The listing builds one solid part. Answer for the finished solid, in the listing's coordinates (mm). A direction names the side the tool comes from. Give positions to 0.01 mm unless a question says otherwise; leave off trailing zeros. Loops run counter-clockwise (first coordinate to the right, second up) from the corner with the lowest first, then second, coordinate; pieces in that order, holes last.
Item 1: Each of these flat-tipped pins is pushed along its axis until it touches: pin 1 Ø4 at (x, z) = (-17.5, -22) entering from +Y; pin 2 Ø1.5 at (x, z) = (7, -1) entering from -Y; pin 3 Ø6 at (x, z) = (-11.5, -0.5) entering from +Y. Where does it stop, or does it pass through?
Item 2: Section B-B, the plane z = -33 is taken. Give the vertices of the cut face in (x, y).
Item 3: A tool of negligible diameter and unlimited length cuts with its end or side. For faces 3 (the face through (-1, 10, -37)), 4 (the face through (38, -4, 29)), 5 (the face through (0.5, 9, -23)), 6 (the face through (39, 6, -33)), 7 (the face through (39, 4, 31)), from which of +Z, -Z, +X, -X, +Y, -Y can it reach the whole face along a straight path? Write none if from no direction.
Item 4: Section A-A, the plane y = 10.5 is taken. Give the number of separate pieces and of enclosed holes in the cut face, and give its area (3 significant figures).
Item 5: The mould has two halves that part along X. Classify faces 1 (the face through (-37, -4, -35)), 2 (the face through (-38.52, -3.93, 31.5)): pulls with the +X half, pulls with the -X half, needs draft (parallel to the pull), parting line crosses it, or undercut.
Item 6: Section D-D, the plane y = 19 is taken. Give the vertices of the cut face in (x, z), and give its area (3 significant figures).
Item 7: Consider line 1 along X through (y, z) = (2.5, 18); line 2 along X through (y, z) = (16.25, 31.5); line 3 along X through (y, z) = (20.25, -8). Determine where each line is inside the solid, lowest interval first.
from build123d import *

# Parameters (mm, degrees)
SKETCH_1_W          = 80
SKETCH_1_H          = 74
EXTRUDE_1_DEPTH     = 2
SKETCH_2_W          = 80
SKETCH_2_H          = 74
SKETCH_2_W_2        = 76
SKETCH_2_H_2        = 70
EXTRUDE_2_DEPTH     = 20
SKETCH_3_W          = 2
SKETCH_3_H          = 4
CUT_EXTRUDE_3_DEPTH = 4
SKETCH_4_W          = 1
SKETCH_4_H          = 16
SKETCH_4_H_2        = 20
EXTRUDE_3_DEPTH     = 15
SKETCH_6_W          = 3
SKETCH_6_H          = 8
EXTRUDE_4_DEPTH     = 8
SKETCH_7_R          = 1.5
CUT_EXTRUDE_5_DEPTH = 91.846023578


with BuildPart() as part:
    # Эскиз1 → Бобышка-Вытянуть1 (new body)
    with BuildSketch(Plane(origin=(0, 0, 0), x_dir=(1, 0, 0), z_dir=(0, 1, 0))):
        Rectangle(SKETCH_1_W, SKETCH_1_H)
    extrude(amount=EXTRUDE_1_DEPTH)

    # Эскиз2 → Бобышка-Вытянуть2 (add)
    with BuildSketch(Plane(origin=(0, 2, 0), x_dir=(1, 0, 0), z_dir=(0, 1, 0))):
        Rectangle(SKETCH_2_W, SKETCH_2_H)
        Rectangle(SKETCH_2_W_2, SKETCH_2_H_2, mode=Mode.SUBTRACT)
    extrude(amount=EXTRUDE_2_DEPTH)

    # Эскиз3 → Вырез-Вытянуть3 (cut)
    with BuildSketch(Plane(origin=(0, 2, 0), x_dir=(1, 0, 0), z_dir=(0, 1, 0))):
        with Locations((-39, 33)):
            Rectangle(SKETCH_3_W, SKETCH_3_H)
        with Locations((39, 33)):
            Rectangle(SKETCH_3_W, SKETCH_3_H)
        with Locations((39, -33)):
            Rectangle(SKETCH_3_W, SKETCH_3_H)
        with Locations((-39, -33)):
            Rectangle(SKETCH_3_W, SKETCH_3_H)
    extrude(amount=CUT_EXTRUDE_3_DEPTH, mode=Mode.SUBTRACT)

    # Эскиз4 → Бобышка-Вытянуть3 (add)
    with BuildSketch(Plane(origin=(0, 2, 0), x_dir=(1, 0, 0), z_dir=(0, 1, 0))):
        with Locations((-19, 23)):
            Rectangle(SKETCH_4_W, SKETCH_4_H)
        with Locations((0, 23)):
            Rectangle(SKETCH_4_W, SKETCH_4_H)
        with Locations((19, 23)):
            Rectangle(SKETCH_4_W, SKETCH_4_H)
        with Locations((-19, -23)):
            Rectangle(SKETCH_4_W, SKETCH_4_H)
        with Locations((0, -23)):
            Rectangle(SKETCH_4_W, SKETCH_4_H)
        with Locations((19, -25)):
            Rectangle(SKETCH_4_W, SKETCH_4_H_2)
    extrude(amount=EXTRUDE_3_DEPTH)

    # Эскиз6 → Бобышка-Вытянуть4 (add)
    with BuildSketch(Plane.XZ):
        with Locations((38.5, 33)):
            Rectangle(SKETCH_6_W, SKETCH_6_H)
        with Locations((38.5, -33)):
            Rectangle(SKETCH_6_W, SKETCH_6_H)
        with Locations((-38.5, -33)):
            Rectangle(SKETCH_6_W, SKETCH_6_H)
        with Locations((-38.5, 33)):
            Rectangle(SKETCH_6_W, SKETCH_6_H)
    extrude(amount=EXTRUDE_4_DEPTH)

    # Эскиз7 → Вырез-Вытянуть5 (cut, through all)
    with BuildSketch(Plane.ZY.offset(40)):
        with Locations((33, -4)):
            Circle(SKETCH_7_R)
        with Locations((-33, -4)):
            Circle(SKETCH_7_R)
    extrude(amount=-CUT_EXTRUDE_5_DEPTH, mode=Mode.SUBTRACT)


solid = part.part
Worked answers:
1. pin 1: stops at y = 17
1. pin 2: stops at y = 0
1. pin 3: stops at y = 2
2. outline: (-40, -8) - (-37, -8) - (-37, -5.5) - (-40, -5.5) - close; (-40, -2.5) - (-37, -2.5) - (-37, 0) - (37, 0) - (37, -2.5) - (40, -2.5) - (40, 2) - (-40, 2) - close; (-40, 6) - (-38, 6) - (-38, 22) - (-40, 22) - close; (37, -8) - (40, -8) - (40, -5.5) - (37, -5.5) - close; (38, 6) - (40, 6) - (40, 22) - (38, 22) - close
3. face 3: -Z, +X, -X, +Y, -Y
3. face 4: +X, -X, -Y
3. face 5: +Y
3. face 6: +X, -X
3. face 7: +X
4. separate pieces: 6
4. enclosed holes: 1
4. area: 700 mm2
5. face 1: undercut
5. face 2: needs draft
6. outline: (-40, -37) - (40, -37) - (40, 37) - (-40, 37) - close; hole (-38, -35) - (38, -35) - (38, 35) - (-38, 35) - close
6. area: 600 mm2
7. line 1: x = -40 to -38, -19.5 to -18.5, -0.5 to 0.5, 18.5 to 19.5, 38 to 40
7. line 2: x = -40 to -38, 18.5 to 19.5, 38 to 40
7. line 3: x = -40 to -38, 38 to 40
